CAD build for the part. Positions are in the model's coordinates, mm. Face numbers are marked on the shaded views. A direction names the side the tool comes from. Give positions to 0.01 mm unless a question says otherwise; leave off trailing zeros. Loops run counter-clockwise (first coordinate to the right, second up) from the corner with the lowest first, then second, coordinate; pieces in that order, holes last. Notation, with made-up numbers: (72, -39) - (120, -39) arc R26 cw to (120, -6) - close; hole circle Ø8 at (-35, 2.5). An arc over 180 degrees is marked (long way). Return JSON: item names as keys, results as strings.
from build123d import *

# Parameters (mm, degrees)
PAD_DEPTH       = 0.4
SKETCH001_R     = 2
POCKET_DEPTH    = 5
PAD001_DEPTH    = 6.15
POCKET001_DEPTH = 6.551
FILLET_R        = 0.5
FILLET001_R     = 0.39
FILLET002_R     = 0.9


with BuildPart() as part:
    # Sketch → Pad (new body)
    with BuildSketch(Plane.XY):
        with BuildLine():
            Line((-32.7, 6.275), (32.7, 6.275))
            ThreePointArc((34.7, 4.275), (34.114214, 5.689214), (32.7, 6.275))
            Line((34.7, 4.275), (34.7, -4.275))
            ThreePointArc((32.7, -6.275), (34.114214, -5.689214), (34.7, -4.275))
            Line((32.7, -6.275), (-32.7, -6.275))
            ThreePointArc((-34.7, -4.275), (-34.114214, -5.689214), (-32.7, -6.275))
            Line((-34.7, -4.275), (-34.7, 4.275))
            ThreePointArc((-32.7, 6.275), (-34.114214, 5.689214), (-34.7, 4.275))
        make_face()
    extrude(amount=PAD_DEPTH)

    # Sketch001 (on Face10 of Pad) → Pocket (cut)
    with BuildSketch(Plane.XY.offset(0.4)):
        with Locations((-31.755, 0)):
            Circle(SKETCH001_R)
        with Locations((31.755, 0)):
            Circle(SKETCH001_R)
    extrude(amount=-POCKET_DEPTH, mode=Mode.SUBTRACT)

    # Sketch002 (on Face5 of Pocket) → Pad001 (join)
    with BuildSketch(Plane.XY.offset(0.4)):
        with BuildLine():
            Line((-24.865, 3.935), (24.865, 3.935))
            ThreePointArc((27.371365, 0.948231), (26.814529, 3.025959), (24.865, 3.935))
            Line((27.371365, 0.948231), (26.881365, -1.831769))
            ThreePointArc((24.375, -3.935), (26.010959, -3.339529), (26.881365, -1.831769))
            Line((24.375, -3.935), (-24.375, -3.935))
            ThreePointArc((-26.881365, -1.831769), (-26.010959, -3.339529), (-24.375, -3.935))
            Line((-26.881365, -1.831769), (-27.371365, 0.948231))
            ThreePointArc((-24.865, 3.935), (-26.814529, 3.025959), (-27.371365, 0.948231))
        make_face()
    extrude(amount=PAD001_DEPTH)

    # Sketch003 (on Face21 of Pad001) → Pocket001 (cut, through all)
    with BuildSketch(Plane.XY.offset(6.55)):
        with BuildLine():
            Line((-24.865, 3.535), (24.865, 3.535))
            ThreePointArc((26.977437, 1.017664), (26.50812, 2.768834), (24.865, 3.535))
            Line((26.977437, 1.017664), (26.487437, -1.762336))
            ThreePointArc((24.375, -3.535), (25.753834, -3.03312), (26.487437, -1.762336))
            Line((24.375, -3.535), (-24.375, -3.535))
            ThreePointArc((-26.487437, -1.762336), (-25.753834, -3.03312), (-24.375, -3.535))
            Line((-26.487437, -1.762336), (-26.977437, 1.017664))
            ThreePointArc((-24.865, 3.535), (-26.50812, 2.768834), (-26.977437, 1.017664))
        make_face()
    extrude(amount=-POCKET001_DEPTH, mode=Mode.SUBTRACT)

    # Fillet
    fillet_edges = [part.edges().sort_by_distance(p)[0] for p in [
        (0, -3.935, 0.4),
    ]]
    fillet(fillet_edges, radius=FILLET_R)

    # Fillet001
    fillet001_edges = [part.edges().sort_by_distance(p)[0] for p in [
        (-26.010959, -3.339529, 6.55),
    ]]
    fillet(fillet001_edges, radius=FILLET001_R)

    # Fillet002
    fillet002_edges = [part.edges().sort_by_distance(p)[0] for p in [
        (0, 3.535, 0),
    ]]
    fillet(fillet002_edges, radius=FILLET002_R)


solid = part.part
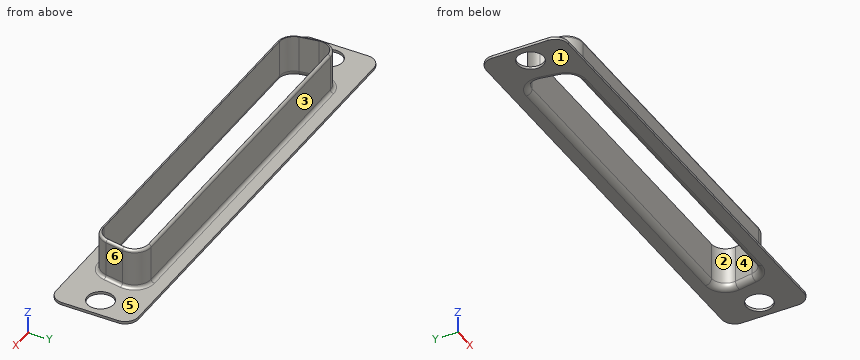
1. Which spindle directions (+Z, -Z, +X, -X, +Y, -Y) get a long thin tool onto all of the face, cutting with end or side? Do the marked faces 4, 5 and 6. Say none if no direction does.
Values follow:
{"face 4": "+Z, -Z", "face 5": "+Z", "face 6": "+Z, +X, -Y"}
2. Drop flat-ended pins along their axis: P1, Ø1.7, axis at x = -2, z = 5, coming from the +Y side (3 decimals); P2, Ø2.5, axis at x = 11.5, z = 4, coming from the -Y side (3 decimals). Give the stop position or say it passes through.
Values follow:
{"P1": "stops at y = 3.935", "P2": "stops at y = -3.935"}
3. Drill centre lines: probe 1 along Y at (x, z) = (-6, 2.75) (3 decimals); probe 2 along X at (y, z) = (1.5, 2.5); probe 3 along Z at (x, y) = (28.5, -5.5). Where is each one in solid material? Low to high.
Values follow:
{"probe 1": "y = -3.935 to -3.535, 3.535 to 3.935", "probe 2": "x = -27.41 to -27.01, 27.01 to 27.41", "probe 3": "z = 0 to 0.4"}
4. Cut at B-B, the plane z = 4.75. Write the cut outline in (x, y) (3 decimals).
Values follow:
{"outline": "(-27.371, 0.948) - (-26.881, -1.832) arc R2.545 ccw to (-24.375, -3.935) - (24.375, -3.935) arc R2.545 ccw to (26.881, -1.832) - (27.371, 0.948) arc R2.545 ccw to (24.865, 3.935) - (-24.865, 3.935) arc R2.545 ccw to start; hole (-26.977, 1.018) - (-26.487, -1.762) arc R2.145 ccw to (-24.375, -3.535) - (24.375, -3.535) arc R2.145 ccw to (26.487, -1.762) - (26.977, 1.018) arc R2.145 ccw to (24.865, 3.535) - (-24.865, 3.535) arc R2.145 ccw to start"}
5. Cut at C-C, the plane y = 0. Give the number of separate pieces and of enclosed holes in the cut face, plus the area to 3 significant figures.
Values follow:
{"separate pieces": "4", "enclosed holes": "0", "area": "7.81 mm²"}
6. Cut at A-A, the plane x = 6.5. Write the cut outline in (y, z) (3 decimals).
Values follow:
{"outline": "(-6.275, 0) - (-4.435, 0) arc R0.9 ccw to (-3.535, 0.9) - (-3.535, 6.55) - (-3.545, 6.55) arc R0.39 ccw to (-3.935, 6.16) - (-3.935, 0.9) arc R0.5 cw to (-4.435, 0.4) - (-6.275, 0.4) - close; (3.535, 0.9) arc R0.9 ccw to (4.435, 0) - (6.275, 0) - (6.275, 0.4) - (4.435, 0.4) arc R0.5 cw to (3.935, 0.9) - (3.935, 6.16) arc R0.39 ccw to (3.545, 6.55) - (3.535, 6.55) - close"}
7. Pull direction Y, two halves, no side cores. Call the marked faces 1, 2 and 3: +Y half, -Y half, draft (parallel to the pull), parting line (faces both ways), or undercut.
Values follow:
{"face 1": "draft", "face 2": "undercut", "face 3": "+Y half"}
